The listing builds one solid part. Answer for the finished solid, in the listing's coordinates (mm). A direction names the side the tool comes from. Round coordinates to 2 decimals unless told otherwise and drop trailing zeros. Loops run counter-clockwise (first coordinate to the right, second up) from the corner with the lowest first, then second, coordinate; pieces in that order, holes last. Notation, with made-up numbers: (-13.75, 62.5) -> (-4.75, 62.5) arc R22 ccw to (-4.75, 91.5) -> close; hole circle Ø7 at (-11.5, 65.25). An arc over 180 degrees is marked (long way). Answer in a Markdown table with one row per item. Add a question column.
```python
from build123d import *

# Parameters (mm, degrees)
CROQUIS1_R              = 1
SALIENTE_EXTRUIR1_DEPTH = 3


with BuildPart() as part:
    # Croquis1 → Saliente-Extruir1 (new body)
    with BuildSketch(Plane.XY):
        with BuildLine():
            Line((28.59683313, -20.934226553), (28.59683313, -14.934226553))
            ThreePointArc((28.59683313, -14.934226553), (42.193666261, 0), (28.59683313, 14.934226553))
            Line((28.59683313, 14.934226553), (28.59683313, 17.934226553))
            Line((28.59683313, 17.934226553), (-1.40316687, 17.934226553))
            Line((-1.40316687, 17.934226553), (-1.40316687, 14.934226553))
            ThreePointArc((-1.40316687, 14.934226553), (-15, 0), (-1.40316687, -14.934226553))
            Line((-1.40316687, -14.934226553), (-1.40316687, -20.934226553))
            Line((-1.40316687, -20.934226553), (28.59683313, -20.934226553))
        make_face()
        with Locations((-7.40316687, 8.867372458)):
            Circle(CROQUIS1_R, mode=Mode.SUBTRACT)
        with Locations((34.59683313, 8.867372458)):
            Circle(CROQUIS1_R, mode=Mode.SUBTRACT)
        with Locations((34.59683313, -8.132627542)):
            Circle(CROQUIS1_R, mode=Mode.SUBTRACT)
        with Locations((-7.40316687, -8.132627542)):
            Circle(CROQUIS1_R, mode=Mode.SUBTRACT)
        with BuildLine():
            Line((0, -10.297541691), (27.193666261, -10.297541691))
            Line((27.193666261, -10.297541691), (27.193666261, -9.297541691))
            ThreePointArc((27.193666261, -9.297541691), (36.491207952, 0), (27.193666261, 9.297541691))
            Line((27.193666261, 9.297541691), (27.193666261, 10.297541691))
            Line((27.193666261, 10.297541691), (0, 10.297541691))
            Line((0, 10.297541691), (0, 9.297541691))
            ThreePointArc((0, 9.297541691), (-9.297541691, 0), (0, -9.297541691))
            Line((0, -9.297541691), (0, -10.297541691))
        make_face(mode=Mode.SUBTRACT)
    extrude(amount=SALIENTE_EXTRUIR1_DEPTH)


solid = part.part
```
Item 1: Section D-D, the plane x = -11 is taken. Write down the section's boundary in (y, z), and give its area (3 significant figures).
Item 2: For faces 4 (the flat face through (14, 10.298, 1)), 5 (the flat face through (-1.403, 16, 1)), 6 (the flat face through (28.597, 16, 1)), 7 (the flat face through (-1.403, -18, 1)), 8 (the flat face through (28.597, -18, 1)), determine the directions among +Z, -Z, +X, -X, +Y, -Y from which every point of the face is accessible in a straight line to the end or side of a thin tool.
Item 3: Consider L1, parallel to X at y = 0.5, z = 2.3; L2, parallel to Y at x = 6.5, z = 1.2; L3, parallel to X at y = 8.5, z = 2.75. Determine where each line is inside the solid, lowest interval first. Write a range as from..to.
Item 4: Section C-C, the plane z = 1.1 is taken. Write down the section's boundary in (x, y).
Item 5: The mould has two halves that part along Y. Classify faces 1 (the cylindrical face through (36.49, -0.2, 1.48)), 2 (the flat face through (13, 12, 0)), 3 (the cylindrical face through (42.19, -0.31, 1.48)): +Y half, -Y half, draft (parallel to the pull), parting line (faces both ways), or undercut.
Item 6: Flat-ended cylindrical pins translate along their axes: P1, Ø0.9, axis at y = -19.5, z = 2, coming from the -X side; P2, Ø0.9, axis at y = 16.5, z = 1.5, coming from the +X side; P3, Ø0.5, axis at y = 10, z = 1.5, coming from the +X side; P4, Ø1.2, axis at x = -7.4, y = 8.87, coming from the +Z side. Find the tip coordinate at first contact, or state that the pin passes through.
Item 7: Section A-A, the plane x = 9.5 is taken. Write down the section's boundary in (y, z).
Item 8: Section B-B, the plane y = 0 is taken. Write down the section's boundary in (x, z), and give its area (3 significant figures).
Here are the results:
| question | item | result |
|---|---|---|
| 1 | outline | (-10.2, 0) -> (10.2, 0) -> (10.2, 3) -> (-10.2, 3) -> close |
| 1 | area | 61.2 mm² |
| 2 | face 4 | +Z, -Z |
| 2 | face 5 | +Z, -Z, -X, +Y |
| 2 | face 6 | +Z, -Z, +X, +Y |
| 2 | face 7 | +Z, -Z, -X, -Y |
| 2 | face 8 | +Z, -Z, +X, -Y |
| 3 | L1 | x = -14.99..-9.28, 36.48..42.19 |
| 3 | L2 | y = -20.93..-10.3, 10.3..17.93 |
| 3 | L3 | x = -12.36..-8.33, -6.47..-3.77, 30.96..33.67, 35.53..39.55 |
| 4 | outline | (-1.4, -20.93) -> (28.6, -20.93) -> (28.6, -14.93) arc R15 ccw to (28.6, 14.93) -> (28.6, 17.93) -> (-1.4, 17.93) -> (-1.4, 14.93) arc R15 ccw to (-1.4, -14.93) -> close; hole circle Ø2 at (-7.4, -8.13); hole circle Ø2 at (-7.4, 8.87); hole (0, -10.3) -> (27.19, -10.3) -> (27.19, -9.3) arc R9.3 ccw to (27.19, 9.3) -> (27.19, 10.3) -> (0, 10.3) -> (0, 9.3) arc R9.3 ccw to (0, -9.3) -> close; hole circle Ø2 at (34.6, -8.13); hole circle Ø2 at (34.6, 8.87) |
| 5 | face 1 | undercut |
| 5 | face 2 | draft |
| 5 | face 3 | parting line |
| 6 | P1 | stops at x = -1.4 |
| 6 | P2 | stops at x = 28.6 |
| 6 | P3 | stops at x = 38.59 |
| 6 | P4 | passes through |
| 7 | outline | (-20.93, 0) -> (-10.3, 0) -> (-10.3, 3) -> (-20.93, 3) -> close; (10.3, 0) -> (17.93, 0) -> (17.93, 3) -> (10.3, 3) -> close |
| 8 | outline | (-15, 0) -> (-9.3, 0) -> (-9.3, 3) -> (-15, 3) -> close; (36.49, 0) -> (42.19, 0) -> (42.19, 3) -> (36.49, 3) -> close |
| 8 | area | 34.2 mm² |
